from build123d import *

# Parameters (mm, degrees)
F1_DEPTH      = 60
F2_W          = 2.3736116251
F2_H          = 5
F2_W_2        = 3.7527767497
F3_DEPTH      = 5
F5_DEPTH      = 4
F7_DEPTH      = 4
F8_W          = 4
F8_H          = 5
F9_DEPTH      = 5
F10_W         = 4
F10_H         = 5
F11_DEPTH     = 5
F12_T4_DEPTH  = 16.3154051471
F12_T9_DEPTH  = 16.3154051471
F13_T1_DEPTH  = 14.0395087016
F13_T3_DEPTH  = 14.0395087016
F13_T5_DEPTH  = 14.0395087016
F13_T7_DEPTH  = 14.0395087016
F13_T9_DEPTH  = 14.0395087016
F13_T14_DEPTH = 14.0395087016
F13_T19_DEPTH = 14.0395087016
F13_T24_DEPTH = 14.0395087016
F13_T29_DEPTH = 14.0395087016


# Not quite as in the source:
# - a fillet or chamfer that OpenCascade refuses, or shapes differently, is made with other operations: its cross-section is extruded or revolved along the edge and cut away or added


with BuildPart() as f1:
    # F0 (on Front) → F1 (new body, symmetric)
    with BuildSketch(Plane.XZ):
        Polygon((1.8763883749, -3.25), (3.7527767497, 0), (1.8763883749, 3.25), (-1.8763883749, 3.25), (-3.7527767497, 0), (-1.8763883749, -3.25), align=None)
    extrude(amount=F1_DEPTH, both=True)

    # F2 (on face) → F3 (join, symmetric)
    with BuildSketch(Plane.XY.offset(3.25)):
        with Locations((-3.0631941874, -55)):
            Rectangle(F2_W, F2_H)
        with Locations((0, -55)):
            Rectangle(F2_W_2, F2_H)
        with Locations((3.0631941874, -55)):
            Rectangle(F2_W, F2_H)
    extrude(amount=F3_DEPTH, both=True)

    # F4 (on face) → F5 (join)
    with BuildSketch(Plane.XZ.offset(57.5)):
        Polygon((-4.25, 8.25), (-4.25, 3.25), (-1.8763883749, 3.25), (1.8763883749, 3.25), (4.25, 3.25), (4.25, 8.25), align=None)
    extrude(amount=F5_DEPTH)

    # F6 (on face) → F7 (join)
    with BuildSketch(Plane(origin=(0, -52.5, 0), x_dir=(-1, 0, 0), z_dir=(0, 1, 0))):
        Polygon((-4.25, 8.25), (-4.25, 3.25), (-1.8763883749, 3.25), (1.8763883749, 3.25), (4.25, 3.25), (4.25, 8.25), align=None)
    extrude(amount=F7_DEPTH)

    # F8 (on face) → F9 (join)
    with BuildSketch(Plane.YZ.offset(4.25)):
        with Locations((-59.5, 5.75)):
            Rectangle(F8_W, F8_H)
        with Locations((-50.5, 5.75)):
            Rectangle(F8_W, F8_H)
    extrude(amount=F9_DEPTH)

    # F10 (on face) → F11 (join)
    with BuildSketch(Plane(origin=(-4.25, 0, 0), x_dir=(0, -1, 0), z_dir=(-1, 0, 0))):
        with Locations((50.5, 5.75)):
            Rectangle(F10_W, F10_H)
        with Locations((59.5, 5.75)):
            Rectangle(F10_W, F10_H)
    extrude(amount=F11_DEPTH)

    # F12: chamfer of 2.2 on 2 edges, made by hand


with BuildPart() as f12_tool2:
    # F12_s3 → F12_t4 (new body)
    with BuildSketch(Plane.XZ.offset(63.1577025735)):
        Polygon((4.25, 0.45), (2.05, -1.75), (4.25, -1.75), align=None)
    extrude(amount=-F12_T4_DEPTH)

    split(bisect_by=Plane(origin=(2.8145825623, 0, -1.625), x_dir=(0, 1, 0), z_dir=(0.8660254038, 0, -0.5)), keep=Keep.TOP)


with BuildPart() as f1_1:
    add(f1.part)

    # F12_t1: cut F12_tool2
    add(f12_tool2.part, mode=Mode.SUBTRACT)


with BuildPart() as f12_tool7:
    # F12_s8 → F12_t9 (new body)
    with BuildSketch(Plane.XZ.offset(46.8422974265)):
        Polygon((-4.25, 0.45), (-2.05, -1.75), (-4.25, -1.75), align=None)
    extrude(amount=F12_T9_DEPTH)

    split(bisect_by=Plane(origin=(-2.8145825623, 0, -1.625), x_dir=(0, 1, 0), z_dir=(-0.8660254038, 0, -0.5)), keep=Keep.TOP)


with BuildPart() as f1_2:
    add(f1_1.part)

    # F12_t6: cut F12_tool7
    add(f12_tool7.part, mode=Mode.SUBTRACT)

    # F13: chamfer of 2 on 11 edges, made by hand

    # F13_s2 → F13_t1 (cut)
    with BuildSketch(Plane(origin=(-3.5098771754, 0, -6.0792855961), x_dir=(0, 1, 0), z_dir=(0.5, 0, 0.8660254038))):
        Polygon((58, -3.25), (60, -1.25), (60, -3.25), align=None)
    extrude(amount=F13_T1_DEPTH, mode=Mode.SUBTRACT)

    # F13_s4 → F13_t3 (cut)
    with BuildSketch(Plane(origin=(3.5098771754, 0, -6.0792855961), x_dir=(0, 1, 0), z_dir=(-0.5, 0, 0.8660254038))):
        Polygon((58, -3.25), (60, -1.25), (60, -3.25), align=None)
    extrude(amount=F13_T3_DEPTH, mode=Mode.SUBTRACT)

    # F13_s6 → F13_t5 (cut)
    with BuildSketch(Plane.YZ.offset(-7.0197543508)):
        Polygon((58, 3.25), (60, 1.25), (60, 3.25), align=None)
        Polygon((60, -1.25), (58, -3.25), (60, -3.25), align=None)
        Polygon((-60, -1.25), (-58, -3.25), (-60, -3.25), align=None)
    extrude(amount=F13_T5_DEPTH, mode=Mode.SUBTRACT)

    # F13_s8 → F13_t7 (cut)
    with BuildSketch(Plane(origin=(3.5098771754, 0, 6.0792855961), x_dir=(0, 1, 0), z_dir=(-0.5, 0, -0.8660254038))):
        Polygon((58, -3.25), (60, -1.25), (60, -3.25), align=None)
    extrude(amount=F13_T7_DEPTH, mode=Mode.SUBTRACT)

    # F13_s10 → F13_t9 (cut)
    with BuildSketch(Plane(origin=(-3.5098771754, 0, 6.0792855961), x_dir=(0, 1, 0), z_dir=(0.5, 0, -0.8660254038))):
        Polygon((58, -3.25), (60, -1.25), (60, -3.25), align=None)
    extrude(amount=F13_T9_DEPTH, mode=Mode.SUBTRACT)


with BuildPart() as f13_tool12:
    # F13_s13 → F13_t14 (new body)
    with BuildSketch(Plane(origin=(-3.5098771754, 0, 6.0792855961), x_dir=(0, 1, 0), z_dir=(0.5, 0, -0.8660254038))):
        Polygon((-60, -1.25), (-58, -3.25), (-60, -3.25), align=None)
    extrude(amount=F13_T14_DEPTH)

    split(bisect_by=Plane.XY.offset(3.25), keep=Keep.BOTTOM)


with BuildPart() as f1_3:
    add(f1_2.part)

    # F13_t11: cut F13_tool12
    add(f13_tool12.part, mode=Mode.SUBTRACT)


with BuildPart() as f13_tool17:
    # F13_s18 → F13_t19 (new body)
    with BuildSketch(Plane(origin=(3.5098771754, 0, 6.0792855961), x_dir=(0, 1, 0), z_dir=(-0.5, 0, -0.8660254038))):
        Polygon((-58, 3.25), (-60, 1.25), (-60, 3.25), align=None)
    extrude(amount=F13_T19_DEPTH)

    split(bisect_by=Plane(origin=(2.8145825623, 0, 1.625), x_dir=(0, 1, 0), z_dir=(-0.8660254038, 0, -0.5)), keep=Keep.TOP)


with BuildPart() as f1_4:
    add(f1_3.part)

    # F13_t16: cut F13_tool17
    add(f13_tool17.part, mode=Mode.SUBTRACT)


with BuildPart() as f13_tool22:
    # F13_s23 → F13_t24 (new body)
    with BuildSketch(Plane(origin=(3.5098771754, 0, -6.0792855961), x_dir=(0, 1, 0), z_dir=(-0.5, 0, 0.8660254038))):
        Polygon((-60, -1.25), (-58, -3.25), (-60, -3.25), align=None)
    extrude(amount=F13_T24_DEPTH)

    split(bisect_by=Plane.XY.offset(3.25), keep=Keep.BOTTOM)


with BuildPart() as f1_5:
    add(f1_4.part)

    # F13_t21: cut F13_tool22
    add(f13_tool22.part, mode=Mode.SUBTRACT)


with BuildPart() as f13_tool27:
    # F13_s28 → F13_t29 (new body)
    with BuildSketch(Plane(origin=(3.5098771754, 0, 6.0792855961), x_dir=(0, 1, 0), z_dir=(-0.5, 0, -0.8660254038))):
        Polygon((-60, -1.25), (-58, -3.25), (-60, -3.25), align=None)
    extrude(amount=F13_T29_DEPTH)

    split(bisect_by=Plane.XY.offset(3.25), keep=Keep.BOTTOM)


with BuildPart() as f1_6:
    add(f1_5.part)

    # F13_t26: cut F13_tool27
    add(f13_tool27.part, mode=Mode.SUBTRACT)


solid = f1_6.part
Design review of the part built by this model. Coordinates are the model's own, in mm. A direction names the side the tool comes from. Round coordinates to 2 decimals unless told otherwise and drop trailing zeros. Loops run counter-clockwise (first coordinate to the right, second up) from the corner with the lowest first, then second, coordinate; pieces in that order, holes last. Notation, with made-up numbers: M -29.75,69 L -1.75,69 A11 ccw -1.75,77 Z; hole C 52,56 d6. An arc over 180 degrees is marked long. Answer as a JSON object with one key per item and string values.
Item 1: Clearance check with flat-ended pins moving along their axes: P1, Ø4, axis at x = 6, z = 4.5, coming from the +Y side; P2, Ø1.2, axis at x = 2.5, z = 1, coming from the -Y side; P3, Ø0.7, axis at x = 2.5, z = 2, coming from the +Y side; P4, Ø5.5, axis at y = -54, z = 3, coming from the -X side. State where each tip first meets the part, or that it passes through.
Answer sheet:
{"P1": "stops at y = -48.5", "P2": "stops at y = -59.18", "P3": "stops at y = 58.43", "P4": "stops at x = -9.25"}
Item 2: Wall thickness on L1, parallel to Y at x = -7, z = 4.5; L2, parallel to Y at x = -3.75, z = 5; L3, parallel to X at y = 24, z = 0: over which ranges is each line inside the solid? List them lowest first. Write a range as from..to.
Answer sheet:
{"L1": "y = -61.5..-57.5, -52.5..-48.5", "L2": "y = -61.5..-48.5", "L3": "x = -3.75..3.75"}
Item 3: We need section A-A on x = -6. Give the boundary of the cut face in (y, z), and give its area (3 significant figures).
Answer sheet:
{"outline": "M -61.5,3.25 L -57.5,3.25 L -57.5,8.25 L -61.5,8.25 Z; M -52.5,3.25 L -48.5,3.25 L -48.5,8.25 L -52.5,8.25 Z", "area": "40.0 mm^2"}
Item 4: We need section C-C on y = -36.5. Give the boundary of the cut face in (x, z), and give its area (3 significant figures).
Answer sheet:
{"outline": "M -3.75,0 L -1.88,-3.25 L 1.88,-3.25 L 3.75,0 L 1.88,3.25 L -1.88,3.25 Z", "area": "36.6 mm^2"}
Item 5: Machinability: for faces 1 (the flat face through (3, -52.5, 2)), 2 (the flat face through (-4.25, -55, 4)), 3 (the flat face through (2.17, 58.76, 1.22)), which of the approach directions +Z, -Z, +X, -X, +Y, -Y give a long, thin tool a straight path to every point of the face, cutting with its end or side? Answer none if there is none.
Answer sheet:
{"face 1": "+X, +Y", "face 2": "+Z, -Z, -X", "face 3": "+Z, +X, +Y"}
Item 6: We need section B-B on z = 4.75. Give the boundary of the cut face in (x, y).
Answer sheet:
{"outline": "M -9.25,-61.5 L 9.25,-61.5 L 9.25,-57.5 L 4.25,-57.5 L 4.25,-52.5 L 9.25,-52.5 L 9.25,-48.5 L -9.25,-48.5 L -9.25,-52.5 L -4.25,-52.5 L -4.25,-57.5 L -9.25,-57.5 Z"}
Item 7: The part is to be moulded in two halves that separate along Z. For faces 4 (the flat face through (-3, -52.5, 2)), 5 (the flat face through (-0.03, 58.79, -2.46)), 6 (the flat face through (4.25, -55, 4)), say which applies: pulls with the +Z half, pulls with the -Z half, needs draft (parallel to the pull), parting line crosses it, or undercut.
Answer sheet:
{"face 4": "undercut", "face 5": "pulls with the -Z half", "face 6": "needs draft"}
